Verification items for the finished model (mm, model axes). A direction names the side the tool comes from. Coordinates: 2 decimals unless noted, no trailing zeros. Order: outer loops, then holes, each group sorted by start corner. A loop starts at its lowest first (then second) coordinate and runs counter-clockwise, first axis right, second up. Notation, with made-up numbers: M 0.25,-10.5 L 51.25,-10.5 A19 ccw 51.25,20.5 Z; hole C 37.25,-11.5 d8. An arc over 180 degrees is marked long. Answer as a JSON object with one key per item and string values. Group by question number.
(1) Access from +Z, -Z, +X, -X, +Y, -Y to the whole of each face (thin tool, end or side, straight path). Record for faces 4 (the face through (-4, 1, -1.473)), 5 (the face through (-4, 2, -15.596)), 6 (the face through (-4, 3.236, -8)).
(2) Cross-section at A-A (y = 0.95). Enter the section's corners in (x, z), plus the area to 3 significant figures.
(3) Material ranges on line 1 (Z direction, x = -4.5, y = 2.05); line 2 (X direction, y = 0.4, z = -6); line 3 (Y direction, x = -4.75, z = -9.5), recorded low to high.
(4) Gauge pin test, flat ends, axial feed: pin 1 Ø0.6 at (x, z) = (-3.5, -3.5) entering from -Y; pin 2 Ø2 at (x, z) = (-4, -11.5) entering from -Y; pin 3 Ø1 at (x, z) = (-4, -7) entering from +Y. Record the tip position at first contact, or that the pin passes through.
(5) Cross-section at B-B (z = -8.25). Enter the section's corners in (x, y), plus the area to 3 significant figures.
(6) Mould release check, pull along X, two halves, no side actions. Record for faces 1 (the face through (-3, 0, -8)), 2 (the face through (-4.43, 4.21, -6.29)), 3 (the face through (-1.473, 1, -8)): released by +X, released by -X, zero draft, split by the parting line, or undercut.
(7) Cross-section at C-C (x = -0.25). Enter the section's corners in (y, z).
(8) Cross-section at D-D (y = 2.9). Enter the section's corners in (x, z), plus the area to 3 significant figures.
Autodesk Inventor part; units mm, degrees
ref_plane "YZ Plane" through (0, 0, 0) normal (1, 0, 0) x (0, 1, 0)
ref_plane "XZ Plane" through (0, 0, 0) normal (0, 1, 0) x (-1, 0, 0)
ref_plane "XY Plane" through (0, 0, 0) normal (0, 0, 1) x (1, 0, 0)
sketch "Sketch1" plane through (0, 0, 0) normal (0, 1, 0) x (-1, 0, 0)
  line L0 (0, 0) -> (7.7978, 0)
  line L1 (7.7978, 0) -> (7.7978, -15.5956)
  line L2 (7.7978, -15.5956) -> (0, -15.5956)
  line L3 (0, -15.5956) -> (0, 0)
  dimension "d0" = 7.7978
  dimension "d1" = 15.5956
extrude "Extrusion1" add sketch "Sketch1" along normal blind 3.236
sketch "Sketch2" plane through (0, 3.236, 0) normal (0, 1, 0) x (1, 0, 0)
  line L0 (0, 0) -> (-3.8989, 0) construction
  line L1 (-3.8989, 0) -> (-3.8989, 3.8989) construction
  line L2 (-3.8989, 3.8989) -> (0, 3.8989) construction
  line L3 (0, 3.8989) -> (0, 0) construction
  circle A0 centre (-3.8989, 3.8989) radius 2.4498
  dimension "d4" = 3.8989
  dimension "d5" = 3.8989
  dimension "d6" = 4.8997
extrude "Extrusion2" add sketch "Sketch2" along normal blind 1.9837
pattern_linear "Rectangular Pattern1" count 2 spacing 7.7978 along (0, 0, -1) of "Extrusion2"
shell "Shell1" thickness 1.4732 removed faces 1 at (-2.5993, 0, -5.1985)
sketch "Sketch3" plane through (-6.3246, 1.7628, -1.4732) normal (0, -1, 0) x (1, 0, 0)
  circle A0 centre (2.4257, -2.4257) radius 2.4498 construction
  circle A1 centre (2.4257, -10.2235) radius 2.4498 construction
  circle A2 centre (2.4257, -2.4257) radius 0.9766 construction
  line L0 (2.4257, -2.4257) -> (2.4257, -10.2235) construction
  circle A3 centre (2.4257, -6.3246) radius 0.6198
  circle A4 centre (2.4257, -6.3246) radius 1.4491
  point P0 (6.3246, 1.4732)
  dimension "d13" = 1.2395
extrude "Extrusion3" add sketch "Sketch3" along normal up to surface (1.7628 mm away)
properties part number "1x2 short orange pegged" material "ABS Plastic"
Taken from the geometry:
{
 "1": {"face 4": "-Y", "face 5": "-Z, +X, -X, +Y, -Y", "face 6": "+Y"},
 "2": {"outline": "M -7.8,-15.6 L 0,-15.6 L 0,0 L -7.8,0 Z; C -3.9,-7.8 d2.9; hole M -6.32,-14.12 L -1.47,-14.12 L -1.47,-1.47 L -6.32,-1.47 Z; hole C -3.9,-7.8 d1.24", "area": "65.6 mm²"},
 "3": {"line 1": "z = -15.6 to -12.47, -10.93 to -4.67, -3.13 to 0", "line 2": "x = -7.8 to -6.32, -1.47 to 0", "line 3": "y = 1.76 to 5.22"},
 "4": {"pin 1": "stops at y = 3.75", "pin 2": "stops at y = 1.76", "pin 3": "stops at y = 3.24"},
 "5": {"outline": "M -7.8,0 L -6.32,0 L -6.32,1.76 L -5.28,1.76 L -5.28,0 L -4.32,0 L -4.32,1.76 L -3.48,1.76 L -3.48,0 L -2.52,0 L -2.52,1.76 L -1.47,1.76 L -1.47,0 L 0,0 L 0,3.24 L -7.8,3.24 Z", "area": "20.0 mm²"},
 "6": {"face 1": "zero draft", "face 2": "split by the parting line", "face 3": "undercut"},
 "7": {"outline": "M 0,-15.6 L 3.24,-15.6 L 3.24,0 L 0,0 Z"},
 "8": {"outline": "M -7.8,-15.6 L 0,-15.6 L 0,0 L -7.8,0 Z; hole C -3.9,-11.7 d1.95; hole C -3.9,-3.9 d1.95", "area": "116 mm²"}
}
